from build123d import *

# Parameters (mm, degrees)
F0_R     = 254
F1_DEPTH = 254


with BuildPart() as f1:
    # F0 (on Front) → F1 (new body)
    with BuildSketch(Plane.XZ):
        with BuildLine():
            ThreePointArc((-227.329998, 127), (-190.13256, 37.197439), (-100.329998, 0))
            Line((-100.329998, 0), (1550.670002, 0))
            Line((1550.670002, 0), (1654.592514, 0))
            Line((1654.592514, 0), (1654.592514, 381))
            Line((1654.592514, 381), (1474.771318, 638.244218))
            Line((1474.771318, 638.244218), (1621.227109, 794.942517))
            Line((1621.227109, 794.942517), (1474.771318, 931.825298))
            Line((1474.771318, 931.825298), (1346.835812, 794.942517))
            Line((1346.835812, 794.942517), (1230.950807, 903.252757))
            Line((1230.950807, 903.252757), (1370.422253, 1052.478254))
            Line((1370.422253, 1052.478254), (1230.950807, 1182.833217))
            Line((1230.950807, 1182.833217), (1057.512871, 997.265756))
            Line((1057.512871, 997.265756), (1057.512871, 1016))
            Line((1057.512871, 1016), (803.512871, 1016))
            Line((803.512871, 1016), (661.670002, 1016))
            Line((661.670002, 1016), (661.670002, 762))
            Line((661.670002, 762), (534.670002, 762))
            Line((534.670002, 762), (534.670002, 1016))
            Line((534.670002, 1016), (153.670002, 1016))
            ThreePointArc((153.670002, 1016), (63.86744, 978.802561), (26.670002, 889))
            Line((26.670002, 889), (26.670002, 508))
            Line((26.670002, 508), (-100.329998, 508))
            ThreePointArc((-100.329998, 508), (-190.13256, 470.802561), (-227.329998, 381))
            Line((-227.329998, 381), (-227.329998, 127))
        make_face()
        with Locations((598.170002, 381)):
            Circle(F0_R, mode=Mode.SUBTRACT)
    extrude(amount=F1_DEPTH)


solid = f1.part
The listing builds one solid part. Answer for the finished solid, in the listing's coordinates (mm). A direction names the side the tool comes from. Coordinates: 2 decimals unless noted, no trailing zeros. Write each loop counter-clockwise with the first axis right and the second up, starting at its lowest first coordinate (ties: lowest second). Pieces come first, ordered by that corner, then holes. Notation, with made-up numbers: (59.25, -22.75) - (107.25, -22.75) arc R28 ccw to (107.25, 14.25) - close; hole circle Ø5 at (9.5, 67). An arc over 180 degrees is marked (long way). Return JSON: item names as keys, results as strings.
1. Which of the six approach directions +Z, -Z, +X, -X, +Y, -Y give full straight-line access (tool end or side, diameter ignored) to faces 4 (the face through (661.67, -125, 891)), 5 (the face through (1299.71, -125.22, 976.82)), 6 (the face through (347, -125, 1016))?
Final values:
{"face 4": "+Z, +Y, -Y", "face 5": "+Y, -Y", "face 6": "+Z, -X, +Y, -Y"}
2. The part is cut by section B-B on z = 598.5. Determine the outline of the cut face in (x, y).
Final values:
{"outline": "(26.67, -254) - (466.98, -254) - (466.98, 0) - (26.67, 0) - close; (729.36, -254) - (1502.55, -254) - (1502.55, 0) - (729.36, 0) - close"}
3. The part is cut by section C-C on z = 444. Determine the outline of the cut face in (x, y), then the cut area to 3 significant figures.
Final values:
{"outline": "(-210.6, -254) - (352.11, -254) - (352.11, 0) - (-210.6, 0) - close; (844.23, -254) - (1610.55, -254) - (1610.55, 0) - (844.23, 0) - close", "area": "338,000 mm^2"}
4. The part is cut by section A-A on y = -134.5. Determine the outline of the cut face in (x, z).
Final values:
{"outline": "(-227.33, 127) arc R127 ccw to (-100.33, 0) - (1654.59, 0) - (1654.59, 381) - (1474.77, 638.24) - (1621.23, 794.94) - (1474.77, 931.83) - (1346.84, 794.94) - (1230.95, 903.25) - (1370.42, 1052.48) - (1230.95, 1182.83) - (1057.51, 997.27) - (1057.51, 1016) - (661.67, 1016) - (661.67, 762) - (534.67, 762) - (534.67, 1016) - (153.67, 1016) arc R127 ccw to (26.67, 889) - (26.67, 508) - (-100.33, 508) arc R127 ccw to (-227.33, 381) - close; hole circle Ø508 at (598.17, 381)"}
5. The part is cut by section D-D on x = 969. Determine the outline of the cut face in (y, z).
Final values:
{"outline": "(-254, 0) - (0, 0) - (0, 1016) - (-254, 1016) - close"}
6. For a pull along Z with two mould halves and no side action, classify faces 1 (the face through (765, -125, 0)), 2 (the face through (1565.94, -125.22, 507.82)), 3 (the face through (1145.4, -125.2, 1091.3)) as +Z half, -Z half, draft (parallel to the pull), parting line (faces both ways), or undercut.
Final values:
{"face 1": "-Z half", "face 2": "undercut", "face 3": "+Z half"}
7. Consider line 1 along Z through (x, y) = (1036, -138); line 2 along X through (y, z) = (-11.5, 232.5); line 3 along X through (y, z) = (-224.5, 785). Determine where each line is inside the solid, lowest interval first.
Final values:
{"line 1": "0 to 1016", "line 2": "-227.33 to 392.1, 804.24 to 1654.59", "line 3": "26.67 to 534.67, 661.67 to 1611.93"}
8. Each of these flat-tipped pins is pushed along its axis until it touches: pin 1 Ø2 at (y, z) = (-124.5, 841) entering from -X; pin 2 Ø10 at (y, z) = (-82, 826.5) entering from +X; pin 3 Ø8 at (y, z) = (-118, 731.5) entering from +X. Where does it stop, or does it pass through?
Final values:
{"pin 1": "x = 26.67", "pin 2": "x = 1592.81", "pin 3": "x = 1565.67"}
